from build123d import *

# Parameters (mm, degrees)
F0_R     = 14.533387
F0_R_2   = 10.506037
F1_DEPTH = 50.8
F0_W     = 81.798442
F0_H     = 78.523383
F2_DEPTH = 25.4
F3_DEPTH = 25.4


with BuildPart() as f1:
    # F0 (on Front) → F1 (new body)
    with BuildSketch(Plane.XZ):
        with Locations((0, -5.688772)):
            Circle(F0_R)
        with Locations((0, -5.688772)):
            Circle(F0_R_2, mode=Mode.SUBTRACT)
    extrude(amount=F1_DEPTH)

    # F0 (on Front) → F2 (join)
    with BuildSketch(Plane.XZ):
        with Locations((1.802664, -5.688772)):
            Rectangle(F0_W, F0_H)
        with Locations((0, -5.688772)):
            Circle(F0_R, mode=Mode.SUBTRACT)
    extrude(amount=F2_DEPTH)

    # F0 (on Front) → F3 (join)
    with BuildSketch(Plane.XZ):
        with Locations((1.802664, -5.688772)):
            Rectangle(F0_W, F0_H)
        with Locations((0, -5.688772)):
            Circle(F0_R, mode=Mode.SUBTRACT)
    extrude(amount=-F3_DEPTH)


solid = f1.part
Build history of the part. All positions in model axes, mm. A direction names the side the tool comes from. Round coordinates to 2 decimals unless told otherwise and drop trailing zeros. Write each loop counter-clockwise with the first axis right and the second up, starting at its lowest first coordinate (ties: lowest second). Pieces come first, ordered by that corner, then holes. Notation, with made-up numbers: (-35, 52) -> (-1, 52) arc R20 ccw to (-1, 66) -> close; hole circle Ø2 at (4.5, -12). An arc over 180 degrees is marked (long way). Write item = value, one per line.
(1) Band-saw the part on B-B (y = -3). Give the cut face in (x, z), then the cut area to 3 significant figures.
Answer:
outline = (-39.1, -44.95) -> (42.7, -44.95) -> (42.7, 33.57) -> (-39.1, 33.57) -> close; hole circle Ø21.01 at (0, -5.69)
area = 6,080 mm2
(2) Band-saw the part on A-A (x = 0). Give the cut face in (y, z), then the cut area to 3 significant figures.
Answer:
outline = (-50.8, -20.22) -> (-25.4, -20.22) -> (-25.4, -44.95) -> (25.4, -44.95) -> (25.4, -20.22) -> (0, -20.22) -> (0, -16.19) -> (-50.8, -16.19) -> close; (-50.8, 4.82) -> (0, 4.82) -> (0, 8.84) -> (25.4, 8.84) -> (25.4, 33.57) -> (-25.4, 33.57) -> (-25.4, 8.84) -> (-50.8, 8.84) -> close
area = 2,920 mm2
(3) Flat gauge pins, fed straight in: pin 1 (1.5 mm diameter, centred on x = -4.5, z = -15, fed in from -Y); pin 2 (8.5 mm diameter, centred on x = -6, z = 0, fed in from +Y). Where does each tip first touch, or does it go through?
Answer:
pin_1 = -50.8
pin_2 = 0
(4) Two-plate mould, pull along Z, no slides. Class faces 4 (the face through (1, 0, 33.573)), 5 (the face through (42.702, 0, -6)), 6 (the face through (-10.496, -25.044, -5.227)): pulls with the +Z half, pulls with the -Z half, needs draft (parallel to the pull), parting line crosses it, or undercut.
Answer:
face_4 = pulls with the +Z half
face_5 = needs draft
face_6 = undercut
(5) Band-saw the part on C-C (z = -27). Give the cut face in (x, y).
Answer:
outline = (-39.1, -25.4) -> (42.7, -25.4) -> (42.7, 25.4) -> (-39.1, 25.4) -> close
(6) Band-saw the part on D-D (x = 32). Give the cut face in (y, z), then the cut area to 3 significant figures.
Answer:
outline = (-25.4, -44.95) -> (25.4, -44.95) -> (25.4, 33.57) -> (-25.4, 33.57) -> close
area = 3,990 mm2
(7) Tool access for faces 1 (the face through (1, 0, -44.95)), 2 (the face through (7.81, -37.92, 6.57)), 3 (the face through (10, 0, -1)): list every direction of +Z, -Z, +X, -X, +Y, -Y with a clear straight run to the whole face (end or side of a thin tool).
Answer:
face_1 = -Z, +X, -X, +Y, -Y
face_2 = -Y
face_3 = +Y
(8) Probe L1, parallel to Z at x = 0, y = -39; L2, parallel to Y at x = -10, z = 10.5; L3, parallel to Z at x = 5, y = -16. List the from-to ranges inside material, lowest first.
Answer:
L1 = -20.22 to -16.19, 4.82 to 8.84
L2 = -25.4 to 25.4
L3 = -44.95 to -14.93, 3.55 to 33.57
